from build123d import *

# Parameters (mm, degrees)
F1_DEPTH = 1.5875
F3_DEPTH = 3.175


with BuildPart() as f1:
    # F0 (on Top) → F1 (new body)
    with BuildSketch(Plane.XY):
        with BuildLine():
            Line((40.410568, 15.044903), (15.010568, 15.044903))
            ThreePointArc((15.010568, 15.044903), (10.52044, 13.185031), (8.660568, 8.694903))
            Line((8.660568, 8.694903), (8.660568, -16.705097))
            ThreePointArc((8.660568, -16.705097), (10.52044, -21.195225), (15.010568, -23.055097))
            Line((15.010568, -23.055097), (40.410568, -23.055097))
            ThreePointArc((40.410568, -23.055097), (44.900696, -21.195225), (46.760568, -16.705097))
            Line((46.760568, -16.705097), (46.760568, 8.694903))
            ThreePointArc((46.760568, 8.694903), (44.900696, 13.185031), (40.410568, 15.044903))
        make_face()
    extrude(amount=F1_DEPTH)

    # F2 (on face) → F3 (join)
    with BuildSketch(Plane.XY.offset(1.5875)):
        with BuildLine():
            ThreePointArc((46.760568, 8.694903), (44.900696, 13.185031), (40.410568, 15.044903))
            Line((40.410568, 15.044903), (15.010568, 15.044903))
            ThreePointArc((15.010568, 15.044903), (10.52044, 13.185031), (8.660568, 8.694903))
            Line((8.660568, 8.694903), (8.660568, -16.705097))
            ThreePointArc((8.660568, -16.705097), (10.52044, -21.195225), (15.010568, -23.055097))
            Line((15.010568, -23.055097), (40.410568, -23.055097))
            ThreePointArc((40.410568, -23.055097), (44.900696, -21.195225), (46.760568, -16.705097))
            Line((46.760568, -16.705097), (46.760568, 8.694903))
        make_face()
        with BuildLine():
            ThreePointArc((10.248068, 7.107403), (12.10794, 11.597531), (16.598068, 13.457403))
            Line((16.598068, 13.457403), (38.823068, 13.457403))
            ThreePointArc((38.823068, 13.457403), (43.313196, 11.597531), (45.173068, 7.107403))
            Line((45.173068, 7.107403), (45.173068, -15.117597))
            ThreePointArc((45.173068, -15.117597), (43.313196, -19.607725), (38.823068, -21.467597))
            Line((38.823068, -21.467597), (16.598068, -21.467597))
            ThreePointArc((16.598068, -21.467597), (12.10794, -19.607725), (10.248068, -15.117597))
            Line((10.248068, -15.117597), (10.248068, 7.107403))
        make_face(mode=Mode.SUBTRACT)
    extrude(amount=-F3_DEPTH)


solid = f1.part
Geometry check sheet. Reference: the model listing, model coordinates, mm. A direction names the side the tool comes from. Round coordinates to 2 decimals unless told otherwise and drop trailing zeros. Order: outer loops, then holes, each group sorted by start corner. A loop starts at its lowest first (then second) coordinate and runs counter-clockwise, first axis right, second up. Notation, with made-up numbers: M 46,-12 L 80,-12 A13 cw 80,8 Z; hole C -39.5,-5.75 d2. An arc over 180 degrees is marked long. Answer in a Markdown table with one row per item. Add a question column.
Item 1: Sectioned sample at A-A, the plane z = -0.8. Enter the section's corners in (x, y), plus the area to 3 significant figures.
Item 2: Draft check along X on faces 1 (the face through (28, -23.055, 0)), 2 (the face through (12.06, 11.55, -0.78)), 3 (the face through (45.173, -4, -1)), 4 (the face through (44.95, 13.135, 0.022)). Enter one of: released by +X, released by -X, zero draft, split by the parting line, or undercut.
Item 3: Sectioned sample at C-C, the plane y = -11. Enter the section's corners in (x, z), plus the area to 3 significant figures.
Item 4: Depth check by flat-ended pin: pin 1 Ø17.5 at (x, y) = (25.5, 2) entering from -Z. Enter the tip coordinate at first touch or a pass-through.
Item 5: Material ranges on L1, parallel to X at y = 6, z = -0.15; L2, parallel to Y at x = 32.5, z = -0.85; L3, parallel to Z at x = 30.5, y = 12, recorded low to high. Write a range as [from, to].
Item 6: Set-up check for faces 5 (the face through (28, 13.457, -1)), 6 (the face through (27, -4, 1.588)): record each of +Z, -Z, +X, -X, +Y, -Y from which the full face is reachable in a straight line by a thin tool's end or side.
Item 7: Sectioned sample at B-B, the plane x = 33.5. Enter the section's corners in (y, z).
Filled in:
| question | item | result |
|---|---|---|
| 1 | outline | M 8.66,-16.71 A6.35 ccw 15.01,-23.06 L 40.41,-23.06 A6.35 ccw 46.76,-16.71 L 46.76,8.69 A6.35 ccw 40.41,15.04 L 15.01,15.04 A6.35 ccw 8.66,8.69 Z; hole M 10.25,-15.12 A6.35 ccw 16.6,-21.47 L 38.82,-21.47 A6.35 ccw 45.17,-15.12 L 45.17,7.11 A6.35 ccw 38.82,13.46 L 16.6,13.46 A6.35 ccw 10.25,7.11 Z |
| 1 | area | 232 mm² |
| 2 | face 1 | zero draft |
| 2 | face 2 | undercut |
| 2 | face 3 | undercut |
| 2 | face 4 | released by +X |
| 3 | outline | M 8.66,-1.59 L 10.25,-1.59 L 10.25,0 L 45.17,0 L 45.17,-1.59 L 46.76,-1.59 L 46.76,1.59 L 8.66,1.59 Z |
| 3 | area | 65.5 mm² |
| 4 | pin 1 | stops at z = 0 |
| 5 | L1 | x = [8.66, 10.25], [45.17, 46.76] |
| 5 | L2 | y = [-23.06, -21.47], [13.46, 15.04] |
| 5 | L3 | z = [0, 1.59] |
| 6 | face 5 | -Z |
| 6 | face 6 | +Z, +X, -X, +Y, -Y |
| 7 | outline | M -23.06,-1.59 L -21.47,-1.59 L -21.47,0 L 13.46,0 L 13.46,-1.59 L 15.04,-1.59 L 15.04,1.59 L -23.06,1.59 Z |
